```python
from build123d import *

# Parameters (mm, degrees)
SKETCH1_R           = 6
BOSS_EXTRUDE1_DEPTH = 6
SKETCH1_3_R         = 3
BOSS_EXTRUDE2_DEPTH = 3
SKETCH2_R           = 3
SKETCH2_R_2         = 1.5
CUT_EXTRUDE1_DEPTH  = 18.23368794


with BuildPart() as part:
    # Sketch1 → Boss-Extrude1 (new body)
    with BuildSketch(Plane(origin=(0, 0, 0), x_dir=(1, 0, 0), z_dir=(0, 1, 0))):
        with Locations(Location((0, 0, 0), (0, 0, 270))):
            Circle(SKETCH1_R)
    extrude(amount=BOSS_EXTRUDE1_DEPTH)

    # Sketch1_3 → Boss-Extrude2 (add)
    with BuildSketch(Plane(origin=(0, 0, 0), x_dir=(1, 0, 0), z_dir=(0, 1, 0))):
        with BuildLine():
            Line((-1.5, 5.809475019), (-12.75, 2.90473751))
            ThreePointArc((-12.75, 2.90473751), (-10.162882693, 2.371708245), (-9, 0))
            ThreePointArc((-9, 0), (-10.162882693, -2.371708245), (-12.75, -2.90473751))
            Line((-12.75, -2.90473751), (-1.5, -5.809475019))
            ThreePointArc((-1.5, -5.809475019), (-6, 0), (-1.5, 5.809475019))
        make_face()
        with Locations((-12, 0)):
            Circle(SKETCH1_3_R)
    extrude(amount=BOSS_EXTRUDE2_DEPTH)

    # Sketch2 → Cut-Extrude1 (cut, through all)
    with BuildSketch(Plane.XZ.offset(-6)):
        with Locations(Location((0, 0, 0), (0, 0, 270))):
            Circle(SKETCH2_R)
        with Locations(Location((-12, 0, 0), (0, 0, 90))):
            Circle(SKETCH2_R_2)
    extrude(amount=CUT_EXTRUDE1_DEPTH, mode=Mode.SUBTRACT)


solid = part.part
```
The model under review builds one solid part; all positions refer to its coordinate system, in mm. A direction names the side the tool comes from. Round coordinates to 2 decimals unless told otherwise and drop trailing zeros. Write each loop counter-clockwise with the first axis right and the second up, starting at its lowest first coordinate (ties: lowest second). Pieces come first, ordered by that corner, then holes. Notation, with made-up numbers: M 85.25,74.5 L 111.25,74.5 A17 ccw 111.25,78.5 Z; hole C -39,-21 d7. An arc over 180 degrees is marked long. Use CSV: the item, a comma, the result in double quotes. Start each with the question number.
(1) We need section A-A, the plane x = 0. State the section outline as (y, z) points, then the cut area to 3 significant figures.
(2) The part is to be moulded in two halves that separate along Z. For faces 1 (the face through (-12.45, 1.52, 1.43)), 2 (the face through (-4, 0, 0)), 3 (the face through (-7.046, 1.479, -4.377)), say which applies: +Z half, -Z half, draft (parallel to the pull), parting line (faces both ways), or undercut.
(3) We need section B-B, the plane z = 0. State the section outline as (x, y) points.
(4) We need section C-C, the plane z = -2. State the section outline as (x, y) points, then the cut area to 3 significant figures.
(5) For line 1 along X through (y, z) = (1.45, 0); line 2 along X through (y, z) = (3.7, 0), list the stretches that pass through material, from the lowest coordinate up.
(6) Tool access review of faces 4 (the face through (3, 6, 1)), 5 (the face through (5.95, 3.62, -0.78)): name each direction out of +Z, -Z, +X, -X, +Y, -Y from which nothing blocks a thin tool from reaching the whole face with its end or side.
(7) We need section D-D, the plane y = 0.45. State the section outline as (x, z) points.
Findings:
1,outline,"M 0,-6 L 6,-6 L 6,-3 L 0,-3 Z; M 0,3 L 6,3 L 6,6 L 0,6 Z"
1,area,"36.0 mm^2"
2,face 1,"undercut"
2,face 2,"draft"
2,face 3,"-Z half"
3,outline,"M -15,0 L -13.5,0 L -13.5,3 L -15,3 Z; M -10.5,0 L -3,0 L -3,6 L -6,6 L -6,3 L -10.5,3 Z; M 3,0 L 6,0 L 6,6 L 3,6 Z"
4,outline,"M -14.24,0 L -2.24,0 L -2.24,6 L -5.66,6 L -5.66,3 L -14.24,3 Z; M 2.24,0 L 5.66,0 L 5.66,6 L 2.24,6 Z"
4,area,"66.8 mm^2"
5,line 1,"-15 to -13.5, -10.5 to -3, 3 to 6"
5,line 2,"-6 to -3, 3 to 6"
6,face 4,"+Z, -Z, +X, -X, +Y"
6,face 5,"+Y"
7,outline,"M -12.75,-2.9 L -1.5,-5.81 A6 ccw long -1.5,5.81 L -12.75,2.9 A3 ccw Z; hole C -12,0 d3; hole C 0,0 d6"
